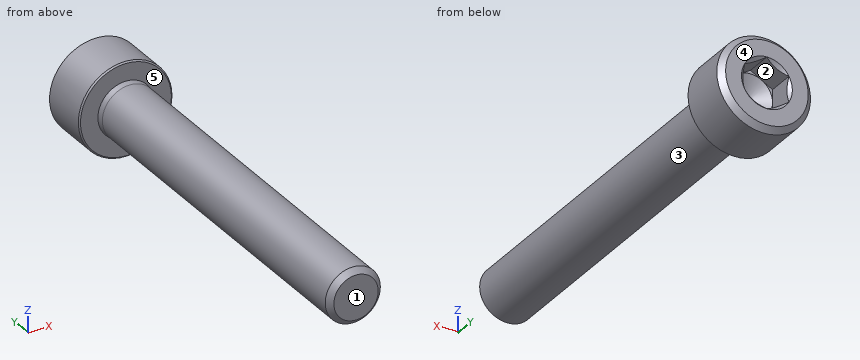
from build123d import *

# Parameters (mm, degrees)
CUT_EXTRUDE1_DEPTH = 2.5


with BuildPart() as part:
    # Sketch1 → Revolve1 (revolve)
    with BuildSketch(Plane.XY):
        Polygon((0, 1.345299462), (2, 2.5), (2, 4.690598923), (2.309401077, 5), (3.75, 5), (4.25, 4.5), (4.25, 0.125), (4.125, 0), (2.55, 0), (2.5, -0.6), (2.5, -34.5095), (2.0095, -35), (0, -35), align=None)
    revolve(axis=Axis((0, -35, 0), (0, 1, 0)))

    # Sketch2 → Cut-Extrude1 (cut)
    with BuildSketch(Plane(origin=(0, 5, 0), x_dir=(1, 0, 0), z_dir=(0, 1, 0))):
        Polygon((-2, -1.154700538), (0, -2.309401077), (2, -1.154700538), (2, 1.154700538), (0, 2.309401077), (-2, 1.154700538), align=None)
    extrude(amount=-CUT_EXTRUDE1_DEPTH, mode=Mode.SUBTRACT)


solid = part.part
Model file for the job. Use its own axes, mm. Face numbers are marked on the shaded views. A direction names the side the tool comes from. Round coordinates to 2 decimals unless told otherwise and drop trailing zeros. Order: outer loops, then holes, each group sorted by start corner. A loop starts at its lowest first (then second) coordinate and runs counter-clockwise, first axis right, second up. Notation, with made-up numbers: M -3,7.25 L 39,7.25 A18 ccw 39,29.25 Z; hole C -5.75,14 d8. An arc over 180 degrees is marked long. Write each question's results on one line, items separated by ' | '. Start each with the question number.
(1) Two-plate mould, pull along Z, no slides. Class the marked faces 1, 2 and 3: pulls with the +Z half, pulls with the -Z half, needs draft (parallel to the pull), parting line crosses it, or undercut.
(2) Saw through at A-A, the plane y = -12. Give the cut face in (x, z).
(3) Probe probe 1 along Y at (x, z) = (3.75, 0.25); probe 2 along Z at (x, y) = (-1.5, -11.5); probe 3 along Z at (x, y) = (1, 1). List the from-to ranges inside material, lowest first. Write a range as from..to.
(4) Which spindle directions (+Z, -Z, +X, -X, +Y, -Y) get a long thin tool onto all of the face, cutting with end or side? Do the marked faces 4 and 5. Say none if no direction does.
(5) Drop flat-ended pins along their axis: pin 1 (2 mm diameter, centred on x = 0.5, y = -27.5, fed in from +Z); pin 2 (1 mm diameter, centred on y = -11, z = -0.5, fed in from -X); pin 3 (3 mm diameter, centred on y = -23.5, z = 0, fed in from +X). Give the stop position or say it passes through.
Established:
1) face 1: needs draft | face 2: undercut | face 3: parting line crosses it
2) outline: C 0,0 d5
3) probe 1: y = 0..4.99 | probe 2: z = -2..2 | probe 3: z = -4.13..4.13
4) face 4: +Z, -Z, +X, -X, +Y | face 5: -Y
5) pin 1: stops at z = 2.5 | pin 2: stops at x = -2.5 | pin 3: stops at x = 2.5
